```python
from build123d import *

# Parameters (mm, degrees)
SKETCH1_W                                      = 112.8
SKETCH1_H                                      = 7
BOSS_EXTRUDE1_DEPTH                            = 7
CSK_FOR_4_FLAT_HEAD_MACHINE_SCREW1_D           = 2.9464
CSK_FOR_4_FLAT_HEAD_MACHINE_SCREW1_CSINK_D     = 7.4535792
CSK_FOR_4_FLAT_HEAD_MACHINE_SCREW1_CSINK_ANGLE = 82
FILLET1_R                                      = 1
SKETCH5_R                                      = 2.325
F_4_40_REGISTRATION_HOLE_DEPTH                 = 2.75


with BuildPart() as part:
    # Sketch1 → Boss-Extrude1 (new body)
    with BuildSketch(Plane(origin=(0, 0, 0), x_dir=(1, 0, 0), z_dir=(0, 1, 0))):
        with Locations((56.4, 3.5)):
            Rectangle(SKETCH1_W, SKETCH1_H)
    extrude(amount=BOSS_EXTRUDE1_DEPTH)

    # CSK for #4 Flat Head Machine Screw1 (through all)
    with Locations(Plane(origin=(0, 0, 0), x_dir=(-1, 0, 0), z_dir=(0, -1, 0))):
        with Locations((-109.4, 3), (-3.4, 3)):
            CounterSinkHole(CSK_FOR_4_FLAT_HEAD_MACHINE_SCREW1_D / 2, CSK_FOR_4_FLAT_HEAD_MACHINE_SCREW1_CSINK_D / 2, counter_sink_angle=CSK_FOR_4_FLAT_HEAD_MACHINE_SCREW1_CSINK_ANGLE)

    # Fillet1
    # the kernel refuses this fillet: 1 mm, written as the material it takes off along each edge
    with BuildSketch(Plane(origin=(0, 0, -9.5), x_dir=(0, 1, 0), z_dir=(0, 0, 1)), Plane(origin=(112.8, 0, -2.026093288), x_dir=(0, 1, 0), z_dir=(0, 0, -1))) as fillet1_piece_1:
        with BuildLine():
            CenterArc((FILLET1_R, -FILLET1_R), FILLET1_R, 90, 90)
            Line((0, -FILLET1_R), (0, 0))
            Line((0, 0), (FILLET1_R, 0))
        make_face()
    extrude(amount=7.473906712, mode=Mode.SUBTRACT)
    with BuildSketch(Plane(origin=(0, 0, -3.973906712), x_dir=(0, 1, 0), z_dir=(0, 0, 1)), Plane(origin=(112.8, 0, 2.5), x_dir=(0, 1, 0), z_dir=(0, 0, -1))) as fillet1_piece_2:
        with BuildLine():
            CenterArc((FILLET1_R, -FILLET1_R), FILLET1_R, 90, 90)
            Line((0, -FILLET1_R), (0, 0))
            Line((0, 0), (FILLET1_R, 0))
        make_face()
    extrude(amount=6.473906712, mode=Mode.SUBTRACT)

    # Sketch5 → 4-40 registration hole (cut)
    with BuildSketch(Plane(origin=(0, 7, 0), x_dir=(1, 0, 0), z_dir=(0, 1, 0))):
        with Locations(Location((3.4, 3, 0), (0, 0, 270))):
            Circle(SKETCH5_R)
    f_4_40_registration_hole = extrude(amount=-F_4_40_REGISTRATION_HOLE_DEPTH, mode=Mode.SUBTRACT)

    # Mirror1: 4-40 registration hole across plane
    add(f_4_40_registration_hole.mirror(Plane(origin=(56.4, 0, 0), x_dir=(0, 0, 1), z_dir=(1, 0, 0))), mode=Mode.SUBTRACT)


solid = part.part
```
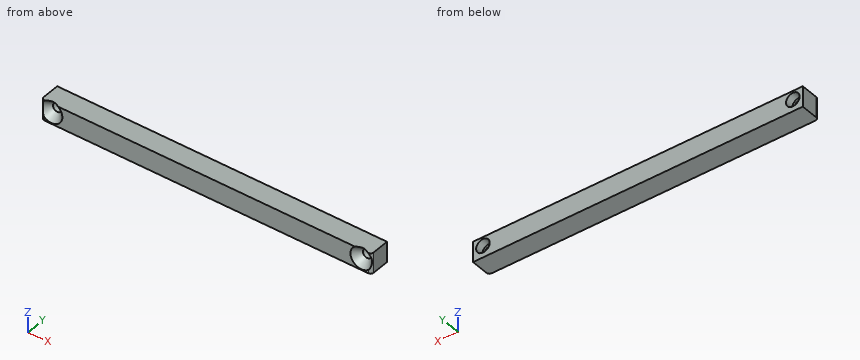
Can you work these out from the model? Positions are in its coordinate system, mm. Coordinates: 2 decimals unless noted, no trailing zeros. Loops run counter-clockwise (first coordinate to the right, second up) from the corner with the lowest first, then second, coordinate; pieces in that order, holes last.
1) Imagine slicing it at A-A on x = 3.4. List the corners of the cut face in (y, z) for me (3 decimals).
2) Imagine slicing it at B-B on z = -3. List the corners of the cut face in (x, y) for me (3 decimals).
3) For pin 1 (4 mm diameter, centred on x = 3.4, z = -3, fed in from +Y); pin 2 (2.5 mm diameter, centred on x = 3.4, z = -3, fed in from +Y), each with a flat end and sliding along its axis, tell me the tip position at first contact or that it passes through.
4) I need wall thicknesses on probe 1 along X at (y, z) = (6.25, -2.75); probe 2 along X at (y, z) = (3.75, -2.75); probe 3 along Z at (x, y) = (3.4, 3.3). Which ranges of each line are inside material? Lowest first, please.
Completed:
1. outline: (0, -7) - (7, -7) - (7, -5.325) - (4.25, -5.325) - (4.25, -4.473) - (2.592, -4.473) - (0, -6.727) - close; (0.836, 0) - (2.592, -1.527) - (4.25, -1.527) - (4.25, -0.675) - (7, -0.675) - (7, 0) - close
2. outline: (0, 1) arc R1 ccw to (0.124, 0.518) - (1.927, 2.592) - (1.927, 4.25) - (1.075, 4.25) - (1.075, 7) - (0, 7) - close; (4.873, 2.592) - (7.127, 0) - (105.673, 0) - (107.927, 2.592) - (107.927, 4.25) - (107.075, 4.25) - (107.075, 7) - (5.725, 7) - (5.725, 4.25) - (4.873, 4.25) - close; (110.873, 2.592) - (112.676, 0.518) arc R1 ccw to (112.8, 1) - (112.8, 7) - (111.725, 7) - (111.725, 4.25) - (110.873, 4.25) - close
3. pin 1: stops at y = 4.25
3. pin 2: passes through
4. probe 1: x = 0 to 1.09, 5.71 to 107.09, 111.71 to 112.8
4. probe 2: x = 0 to 1.95, 4.85 to 107.95, 110.85 to 112.8
4. probe 3: z = -7 to -4.47, -1.53 to 0
